CAD build for the part. Positions are in the model's coordinates, mm. Face numbers are marked on the shaded views. Round coordinates to 2 decimals unless told otherwise and drop trailing zeros. Order: outer loops, then holes, each group sorted by start corner. A loop starts at its lowest first (then second) coordinate and runs counter-clockwise, first axis right, second up. Notation, with made-up numbers: M 42.5,5 L 90.5,5 A16 cw 90.5,26 Z; hole C -33,29 d11. An arc over 180 degrees is marked long. Put each result on its own line as item: value.
Autodesk Inventor part; units mm, degrees
ref_plane "YZ Plane" through (0, 0, 0) normal (1, 0, 0) x (0, 1, 0)
ref_plane "XZ Plane" through (0, 0, 0) normal (0, 1, 0) x (-1, 0, 0)
ref_plane "XY Plane" through (0, 0, 0) normal (0, 0, 1) x (1, 0, 0)
sketch "Sketch1" plane through (0, 0, 0) normal (0, 1, 0) x (-1, 0, 0)
  circle A0 centre (0, 0) radius 1.5
  line L0 (-0.25, 1.479) -> (-0.25, -1.479)
  line L1 (0.25, 1.479) -> (0.25, -1.479)
  line L2 (0, -7.0882) -> (0, 2.9314)
  point P0 (-1.4457, -0.4)
  point P1 (1.4457, -0.4)
  point P2 (1.4967, 0.1)
  point P3 (-1.4967, 0.1)
  dimension "d0" = 3
  dimension "d21" = 0.5
  dimension "d23" = 0.25
extrude "Extrusion1" add sketch "Sketch1" along normal blind 4
extrude "Extrusion2" cut sketch "Sketch1" along normal blind 2.6 contours L1 A0 L2 | L2 A0 L0
sketch "Sketch2" plane through (0, 4, 0) normal (0, 1, 0) x (1, 0, 0)
  line L0 (0, 0) -> (-5.6569, -5.6569)
  line L1 (0, 0) -> (8, 0) construction
  line L2 (0, 0) -> (5.6569, 5.6569)
  line L3 (-5.6569, -5.6569) -> (-9.381, -1.9327)
  line L4 (-9.381, -1.9327) -> (1.9327, 9.381)
  line L5 (1.9327, 9.381) -> (5.6569, 5.6569)
  line L6 (-2.4034, -2.4034) -> (-6.1275, 1.3208)
  line L7 (-2.2144, -2.2144) -> (-5.9386, 1.5097)
  line L8 (-2.2144, -2.2144) -> (1.9327, 1.9327)
  line L9 (1.9327, 1.9327) -> (-1.7914, 5.6569)
  line L10 (1.9327, 1.9327) -> (2.1215, 2.1215)
  line L11 (2.1215, 2.1215) -> (-1.6026, 5.8457)
  dimension "d7" = 8
  dimension "d8" = 135
  dimension "d9" = 8
  dimension "d13" = 0.267
extrude "Extrusion3" add sketch "Sketch1" against normal blind 3.5 contours A0 L1 | L0 A0
revolve "Revolution1" add sketch "Sketch2" angle 360 about axis through (0, 4, 0) along (0.7071, 0, -0.7071)
revolve "Revolution2" cut sketch "Sketch2" angle 360 about axis through (0, 4, 0) along (-0.7071, 0, 0.7071) contours L0 L6 L4 L7
revolve "Revolution3" cut sketch "Sketch2" angle 360 about axis through (0, 4, 0) along (0.7071, 0, -0.7071) contours L9 L4 L11 L2
sketch "Sketch3" plane through (-5.6569, 4, 5.6569) normal (-0.7071, 0, 0.7071) x (0.7071, 0, 0.7071)
  circle A0 centre (0, 0) radius 2.75
  point P0 (0, -4)
  dimension "d16" = 5.5
extrude "Extrusion4" add sketch "Sketch3" along normal blind 2 and the other way blind 16.5
sketch "Sketch5" plane through (0, 0, 0) normal (1, 0, 0) x (0, 1, 0)
  point P0 (0, 0)
sketch "Sketch6" plane through (5.6569, 4, -5.6569) normal (0.7071, 0, -0.7071) x (-0.7071, 0, -0.7071)
  point P0 (0, -4)
properties part number "McCrea_rameno_Walle"
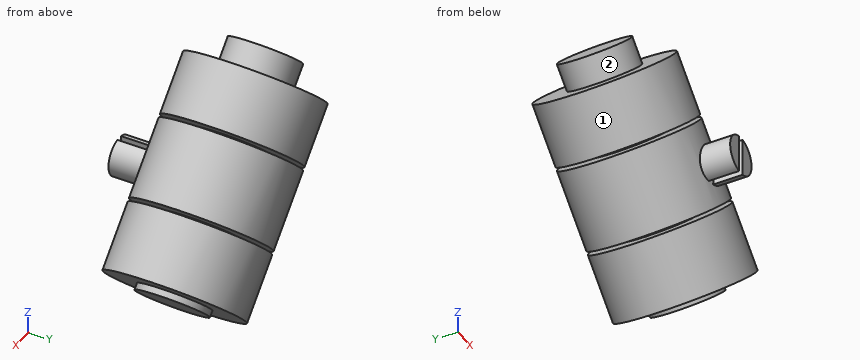
Item 1: Band-saw the part on B-B on y = 7. State how many separate pieces and enclosed holes the cut face has, and give its area (3 significant figures).
Answers below:
separate pieces: 3
enclosed holes: 0
area: 134 mm²
Item 2: Band-saw the part on A-A on y = -2. Give the cut face in (x, z).
Answers below:
outline: M -0.25,-1.48 L -0.25,1.48 A1.5 ccw Z; M 0.25,-1.48 A1.5 ccw 0.25,1.48 Z
Item 3: Probe line 1 along Z through (x, y) = (-0.25, 2.75); line 2 along X through (y, z) = (1, 0.75); line 3 along Y through (x, z) = (5.25, -5). List the from-to ranges inside material, lowest first. Write a range as [from, to].
Answers below:
line 1: [-6.99, -4.49], [-4.12, 4.18], [4.56, 7.49]
line 2: [-6.87, -4.06], [-3.68, 4.62], [4.99, 5.37]
line 3: [-1.26, 9.26]
Item 4: Mould opens along X. For the marked faces 1 and 2 say: pulls with the +X half, pulls with the -X half, needs draft (parallel to the pull), parting line crosses it, or undercut.
Answers below:
face 1: parting line crosses it
face 2: undercut
Item 5: Pin check, flat tips, straight feed: P1, Ø5, axis at y = 5.5, z = 5, coming from the -X side; P2, Ø3, axis at x = 6.5, y = -1, coming from the -Z side; P3, Ø2, axis at y = 3, z = 1, coming from the +X side. Stop position of each tip, or through.
Answers below:
P1: x = -9.02
P2: z = -6.31
P3: x = 7.34
